Can you work these out from the drawing? Everything is in mm from the part's minimum corner. A direction names the side the tool comes from. Round coordinates to 2 decimals unless told otherwise and drop trailing zeros. Write each loop counter-clockwise with the first axis right and the second up, starting at its lowest first coordinate (ties: lowest second). Pieces come first, ordered by that corner, then holes. Notation, with made-up numbers: (60.5, 36.25) - (73.5, 36.25) arc R19 ccw to (73.5, 57.25) - close; hole circle Ø6 at (22.25, 64). An arc over 180 degrees is marked (long way). One line per item, written item: value. Start each with the question number.
(1) On a 3-axis mill with a long thin cutter (end or side, diameter ignored), from which of +Z, -Z, +X, -X, +Y, -Y can I reach the whole of each face in a straight line? I mean the marked faces 1, 2, 3, 4 and 5. Say none if no direction works.
(2) I want a section at D-D on y = 35.5. List the corners of the cut face in (x, z) for me.
(3) I'm going to push flat-ended pins straight in: pin 1 Ø2 at (x, y) = (20, 46.5) entering from +Z; pin 2 Ø3 at (x, z) = (11, 31.5) entering from -Y; pin 3 Ø1.6 at (x, z) = (10.75, 31.92) entering from +Y; pin 4 Ø11 at (x, z) = (9.5, 20.5) entering from +Y. Where does each tip first touch, or does it pass through?
(4) I want a section at B-B on y = 11. List the corners of the cut face in (x, z) for me, plus the area to 3 significant figures.
(5) If I drill on L1, parallel to X at y = 23.7, z = 18.5 (1 decimal); L2, parallel to Z at x = 10, y = 22 (1 decimal); L3, parallel to X at y = 22, z = 18, over which ranges is the centre line in solid material (lowest first)? Write a range as from..to.
(6) I want a section at A-A on z = 27. List the corners of the cut face in (x, y) for me, plus the area to 3 significant figures.
(7) I want a section at C-C on x = 3. List the corners of the cut face in (y, z) for me (1 decimal), plus the area to 3 significant figures.
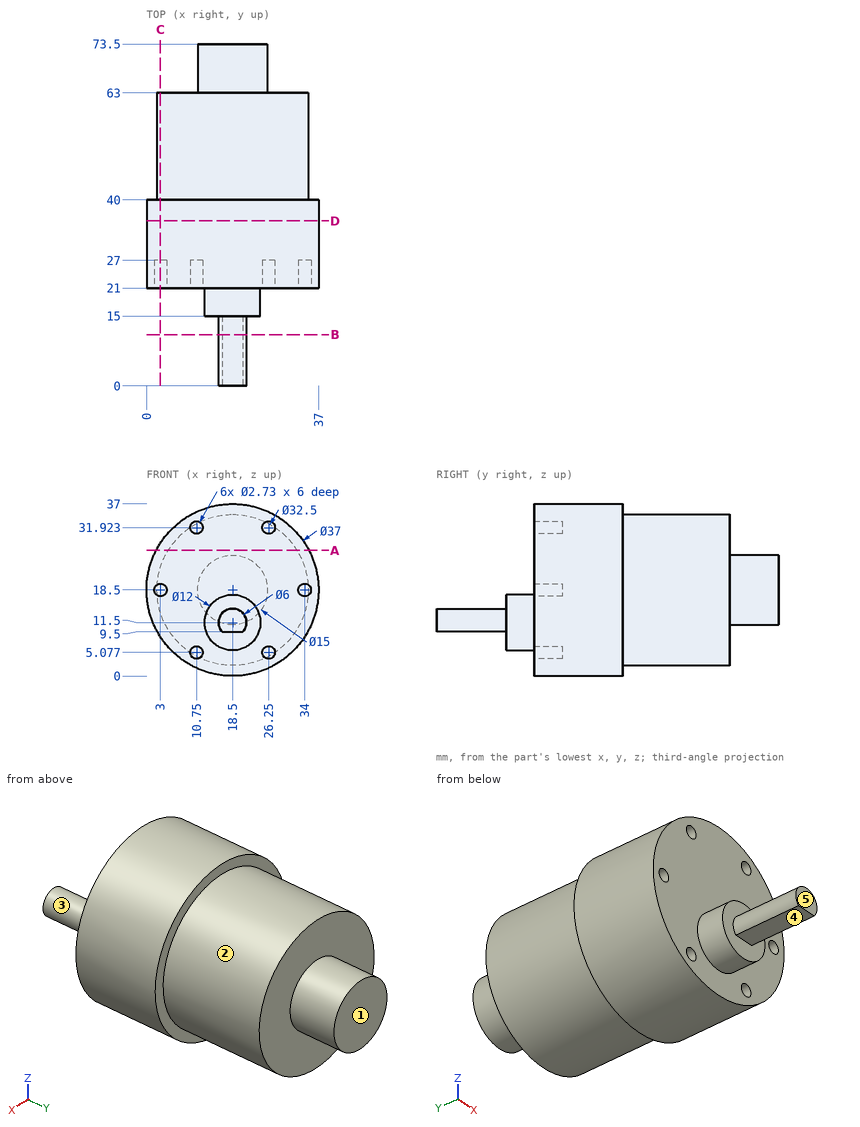
Established:
1. face 1: +Z, -Z, +X, -X, +Y
1. face 2: +Y
1. face 3: -Y
1. face 4: -Z, +X, -X, -Y
1. face 5: +Z, -Z, +X, -X, -Y
2. outline: circle Ø37 at (18.5, 18.5)
3. pin 1: z = 34.74
3. pin 2: y = 21
3. pin 3: y = 63
3. pin 4: y = 73.5
4. outline: (16.26, 9.5) - (20.74, 9.5) arc R3 ccw (long way) to start
4. area: 25.2 mm2
5. L1: 0..1.6, 4.4..32.6, 35.4..37
5. L2: 2.1..3.9, 6.2..30.8, 33.1..34.9
5. L3: 0.01..1.73, 4.27..32.73, 35.27..36.99
6. outline: (2.07, 21) - (34.93, 21) - (34.93, 40) - (32.35, 40) - (32.35, 63) - (4.65, 63) - (4.65, 40) - (2.07, 40) - close
6. area: 1,260 mm2
7. outline: (21, 8.4) - (40, 8.4) - (40, 13.6) - (63, 13.6) - (63, 23.4) - (40, 23.4) - (40, 28.6) - (21, 28.6) - (21, 19.9) - (27, 19.9) - (27, 17.1) - (21, 17.1) - close
7. area: 592 mm2
